Verification items for this drawing (mm, ordinates from the low corner). A direction names the side the tool comes from. Round coordinates to 2 decimals unless told otherwise and drop trailing zeros. Write each loop counter-clockwise with the first axis right and the second up, starting at its lowest first coordinate (ties: lowest second). Pieces come first, ordered by that corner, then holes. Notation, with made-up numbers: M 45.25,80.5 L 75.25,80.5 A20 cw 75.25,94.5 Z; hole C -4.5,-22.5 d9. An arc over 180 degrees is marked long. Write each question's results on one line, items separated by ' | '.
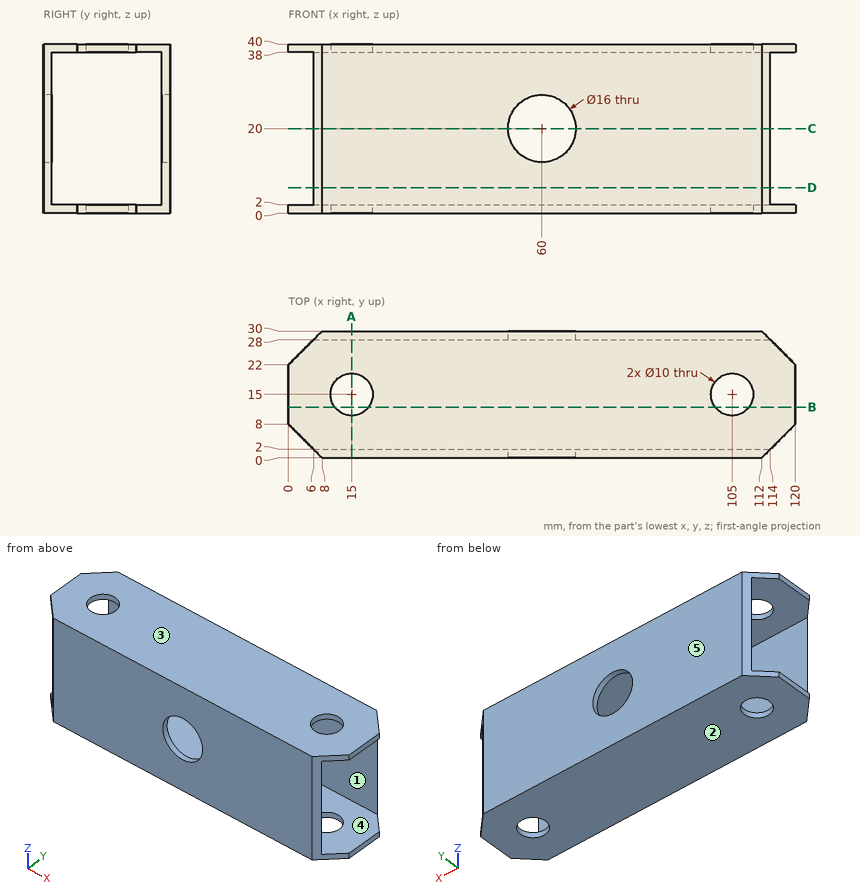
1) Draft check along Z on the marked faces 3, 4 and 5. Enter one of: pulls with the +Z half, pulls with the -Z half, needs draft (parallel to the pull), parting line crosses it, or undercut.
Calculated:
face 3: pulls with the +Z half | face 4: undercut | face 5: needs draft
2) Sectioned sample at D-D, the plane z = 6. Record the cut outline in (x, y), and give its area (3 significant figures).
Calculated:
outline: M 6,2 L 8,0 L 112,0 L 114,2 Z; M 6,28 L 114,28 L 112,30 L 8,30 Z | area: 424 mm²
3) Sectioned sample at A-A, the plane x = 15. Record the cut outline in (y, z), and give its area (3 significant figures).
Calculated:
outline: M 0,0 L 10,0 L 10,2 L 2,2 L 2,38 L 10,38 L 10,40 L 0,40 Z; M 20,0 L 30,0 L 30,40 L 20,40 L 20,38 L 28,38 L 28,2 L 20,2 Z | area: 224 mm²
4) Depth check by flat-ended pin: P1, Ø10, axis at y = 25, z = 9, coming from the -X side. Enter the tip coordinate at first touch or a pass-through.
Calculated:
P1: stops at x = 6
5) Sectioned sample at B-B, the plane y = 12. Record the cut outline in (x, z).
Calculated:
outline: M 0,0 L 11,0 L 11,2 L 0,2 Z; M 0,38 L 11,38 L 11,40 L 0,40 Z; M 19,0 L 101,0 L 101,2 L 19,2 Z; M 19,38 L 101,38 L 101,40 L 19,40 Z; M 109,0 L 120,0 L 120,2 L 109,2 Z; M 109,38 L 120,38 L 120,40 L 109,40 Z
6) Sectioned sample at C-C, the plane z = 20. Record the cut outline in (x, y), and give its area (3 significant figures).
Calculated:
outline: M 6,2 L 8,0 L 52,0 L 52,2 Z; M 6,28 L 52,28 L 52,30 L 8,30 Z; M 68,0 L 112,0 L 114,2 L 68,2 Z; M 68,28 L 114,28 L 112,30 L 68,30 Z | area: 360 mm²
7) Access from +Z, -Z, +X, -X, +Y, -Y to the whole of each face (thin tool, end or side, straight path). Record for the marked faces 1 and 2.
Calculated:
face 1: +X, -X | face 2: -Z, +X, -X, +Y, -Y
8) Material ranges on line 1 (Z direction, x = 108.5, y = 7); line 2 (Y direction, x = 15, z = 0.8); line 3 (Y direction, x = 10.5, z = 35.5), recorded low to high. Write a range as [from, to].
Calculated:
line 1: z = [0, 2], [38, 40] | line 2: y = [0, 10], [20, 30] | line 3: y = [0, 2], [28, 30]
